from build123d import *

# Parameters (mm, degrees)
SKETCH1_W           = 12.7
SKETCH1_H           = 25.4
SKETCH1_R           = 1.4605
BOSS_EXTRUDE1_DEPTH = 2.9718
SKETCH2_W           = 2.9718
SKETCH2_H           = 6.35
CUT_EXTRUDE1_DEPTH  = 15.506691395
FILLET3_R           = 6.35


with BuildPart() as part:
    # Sketch1 → Boss-Extrude1 (new body)
    with BuildSketch(Plane.YZ):
        Rectangle(SKETCH1_W, SKETCH1_H)
        with Locations(Location((0, 6.35, 0), (0, 0, 270))):
            Circle(SKETCH1_R, mode=Mode.SUBTRACT)
    extrude(amount=BOSS_EXTRUDE1_DEPTH)

    # Sketch2 → Cut-Extrude1 (cut, through all)
    with BuildSketch(Plane.YZ.offset(2.9718)):
        with Locations((0.037070408, -9.525)):
            Rectangle(SKETCH2_W, SKETCH2_H)
    extrude(amount=-CUT_EXTRUDE1_DEPTH, mode=Mode.SUBTRACT)

    # Fillet3
    fillet3_edges = [part.edges().sort_by_distance(p)[0] for p in [
        (1.4859, -6.35, 12.7),
        (1.4859, 6.35, 12.7),
    ]]
    fillet(fillet3_edges, radius=FILLET3_R - 0.0001)  # a hair under: the kernel refuses the full size


solid = part.part
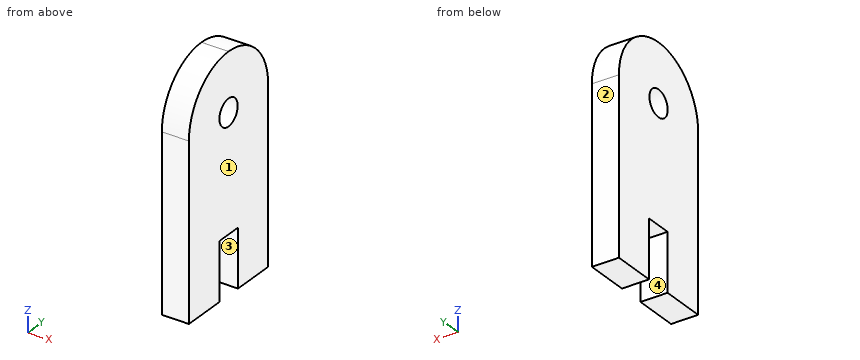
Read the model definition and answer for the solid it produces. Units are mm, in the model's axes. Face numbers are marked on the shaded views. Coordinates: 2 decimals unless noted, no trailing zeros. Order: outer loops, then holes, each group sorted by start corner. A loop starts at its lowest first (then second) coordinate and runs counter-clockwise, first axis right, second up. Notation, with made-up numbers: M 36,41 L 81,41 A22 cw 81,58 Z; hole C 83.25,2.25 d6. An arc over 180 degrees is marked long. Put each result on its own line as item: value. Start each with the question number.
Item 1: The mould has two halves that part along Y. Classify the marked faces 1, 2, 3 and 4: +Y half, -Y half, draft (parallel to the pull), parting line (faces both ways), or undercut.
Item 2: Section C-C, the plane y = 0.25 is taken. Determine the outline of the cut face in (x, z), plus the area to 3 significant figures.
Item 3: Consider probe 1 along Y at (x, z) = (2.35, 6.35); probe 2 along Y at (x, z) = (0.8, 7.5); probe 3 along Z at (x, y) = (2.85, 0.5). Determine where each line is inside the solid, lowest interval first. Write a range as [from, to].
Item 4: Section D-D, the plane y = 3.75 is taken. Determine the outline of the cut face in (x, z), plus the area to 3 significant figures.
Item 5: Given pin 1 Ø0.9 at (x, y) = (1.5, -0.5) entering from -Z, flat-ended and moving along its own axis, determine where the tip first touches the part or whether it passes through.
Item 6: Section A-A, the plane z = -7.75 is taken. Determine the outline of the cut face in (x, y), plus the area to 3 significant figures.
Computed:
1. face 1: draft
1. face 2: +Y half
1. face 3: undercut
1. face 4: undercut
2. outline: M 0,-6.35 L 2.97,-6.35 L 2.97,4.91 L 0,4.91 Z; M 0,7.79 L 2.97,7.79 L 2.97,12.7 L 0,12.7 Z
2. area: 48.0 mm2
3. probe 1: y = [-6.35, -1.46], [1.46, 6.35]
3. probe 2: y = [-6.25, -0.9], [0.9, 6.25]
3. probe 3: z = [-6.35, 4.98], [7.72, 12.68]
4. outline: M 0,-12.7 L 2.97,-12.7 L 2.97,11.47 L 0,11.47 Z
4. area: 71.8 mm2
5. pin 1: stops at z = -6.35
6. outline: M 0,-6.35 L 2.97,-6.35 L 2.97,-1.45 L 0,-1.45 Z; M 0,1.52 L 2.97,1.52 L 2.97,6.35 L 0,6.35 Z
6. area: 28.9 mm2
